Could you check a few things on this model? Use its own coordinates, in mm. A direction names the side the tool comes from. Round coordinates to 2 decimals unless told otherwise and drop trailing zeros. Loops run counter-clockwise (first coordinate to the right, second up) from the corner with the lowest first, then second, coordinate; pieces in that order, holes last. Notation, with made-up numbers: (-20.75, 39) - (-1.75, 39) arc R5 cw to (-1.75, 44) - close; hole circle Ø11 at (46.25, 42). An arc over 180 degrees is marked (long way). Answer as CSV lines item,"result". Start each with the question number.
1) Suppose I cut it at A-A, the plane y = 0.75. Write out the boundary of the cut face in (x, z), then the cut area to 3 significant figures.
2) We'd pull the mould along Z, two halves only. Please class faces 4 (the face through (-1.515, 3.301, 2.597)), 5 (the face through (0, 4, -2.85)), 6 (the face through (-3.25, 5, 0)), 7 (the face through (-3.496, 3.285, 2.049)): pulls with the +Z half, pulls with the -Z half, needs draft (parallel to the pull), parting line crosses it, or undercut.
3) Suppose I cut it at B-B, the plane y = -1. Write out the boundary of the cut face in (x, z).
4) Suppose I cut it at C-C, the plane x = 2.5. Write out the boundary of the cut face in (y, z), then the cut area to 3 significant figures.
5) Suppose I cut it at D-D, the plane z = -0.4. Write out the boundary of the cut face in (x, y), then the cut area to 3 significant figures.
6) Which directions (+Z, -Z, +X, -X, +Y, -Y) give clear straight access to the entire face, cutting with the end or side of a thin tool? Please do faces 1 (the face through (3.504, 3.285, 2.049)), 2 (the face through (0, 2, 0)), 3 (the face through (0.57, 0.5, 0)).
7) I'm going to push flat-ended pins straight in: pin 1 Ø1 at (x, z) = (-0.5, 2.5) entering from +Y; pin 2 Ø0.8 at (x, y) = (1, -1.5) entering from -Z; pin 3 Ø0.8 at (y, z) = (-0.5, 0.5) entering from -X; pin 4 Ø1.5 at (x, z) = (-1.5, 2) entering from +Y. Where does each tip first touch, or does it pass through?
8) Please list where these lines run through material, in increasing order: line 1 along X through (y, z) = (0.25, -2.2); line 2 along Z through (x, y) = (-2.75, 5); line 3 along X through (y, z) = (4.75, -2.1).
```python
from build123d import *
from OCP.BRepFilletAPI import BRepFilletAPI_MakeChamfer

# Parameters (mm, degrees)
CROQUIS2_W              = 7.5
CROQUIS2_H              = 5.7
SALIENTE_EXTRUIR1_DEPTH = 7.2
CROQUIS3_W              = 6.5
CROQUIS3_H              = 4.7
CORTAR_EXTRUIR1_DEPTH   = 5.2
CROQUIS4_W              = 3.6
CROQUIS4_H              = 0.5
CORTAR_EXTRUIR2_DEPTH   = 4.2
CROQUIS5_W              = 1
CROQUIS5_H              = 4.2
CORTAR_EXTRUIR3_DEPTH   = 11.780190165
REDONDEO1_R             = 1
CROQUIS7_W              = 1.4
CROQUIS7_H              = 5.7
CORTAR_EXTRUIR4_DEPTH   = 1
SALIENTE_EXTRUIR2_START = -7.2
CROQUIS6_W              = 0.7
CROQUIS6_H              = 0.7
SALIENTE_EXTRUIR2_DEPTH = 10.7
CHAFL_N1_SIZE           = 0.4
CHAFL_N1_SIZE2          = 0.107179677
CHAFL_N2_SIZE           = 0.4
CHAFL_N2_SIZE2          = 0.107179677
CHAFL_N3_SIZE           = 0.4
CHAFL_N3_SIZE2          = 0.107179677


with BuildPart() as part:
    # Croquis2 → Saliente-Extruir1 (new body)
    with BuildSketch(Plane(origin=(0, 0, 0), x_dir=(1, 0, 0), z_dir=(0, 1, 0))):
        Rectangle(CROQUIS2_W, CROQUIS2_H)
    extrude(amount=SALIENTE_EXTRUIR1_DEPTH)

    # Croquis3 → Cortar-Extruir1 (cut)
    with BuildSketch(Plane(origin=(0, 7.2, 0), x_dir=(1, 0, 0), z_dir=(0, 1, 0))):
        Rectangle(CROQUIS3_W, CROQUIS3_H)
    extrude(amount=-CORTAR_EXTRUIR1_DEPTH, mode=Mode.SUBTRACT)

    # Croquis4 → Cortar-Extruir2 (cut)
    with BuildSketch(Plane(origin=(0, 7.2, 0), x_dir=(1, 0, 0), z_dir=(0, 1, 0))):
        with Locations((0, -2.6)):
            Rectangle(CROQUIS4_W, CROQUIS4_H)
    extrude(amount=-CORTAR_EXTRUIR2_DEPTH, mode=Mode.SUBTRACT)

    # Croquis5 → Cortar-Extruir3 (cut, through all)
    with BuildSketch(Plane(origin=(3.75, 0, 0), x_dir=(0, 0, -1), z_dir=(1, 0, 0))):
        with Locations((-1.85, 5.1)):
            Rectangle(CROQUIS5_W, CROQUIS5_H)
    extrude(amount=-CORTAR_EXTRUIR3_DEPTH, mode=Mode.SUBTRACT)

    # Redondeo1
    # the kernel refuses this fillet: 1 mm, written as the material it adds along each edge
    with BuildSketch(Plane(origin=(1.8, 3, 2.85), x_dir=(0, 1, 0), z_dir=(0, 0, -1)), Plane(origin=(3.75, 3, 2.35), x_dir=(0, 0, -1), z_dir=(-1, 0, 0))) as redondeo1_piece_1:
        with BuildLine():
            CenterArc((REDONDEO1_R, -REDONDEO1_R), REDONDEO1_R, 90, 90)
            Line((0, -REDONDEO1_R), (0, 0))
            Line((0, 0), (REDONDEO1_R, 0))
        make_face()
    extrude(amount=0.5)
    with BuildSketch(Plane(origin=(-1.8, 3, 2.35), x_dir=(1, 0, 0), z_dir=(0, 0, 1)), Plane(origin=(-3.25, 3, 2.35), x_dir=(0, 1, 0), z_dir=(-1, 0, 0))) as redondeo1_piece_2:
        with BuildLine():
            CenterArc((REDONDEO1_R, REDONDEO1_R), REDONDEO1_R, 180, 90)
            Line((0, REDONDEO1_R), (0, 0))
            Line((0, 0), (REDONDEO1_R, 0))
        make_face()
    extrude(amount=0.5)

    # Croquis7 → Cortar-Extruir4 (cut)
    with BuildSketch(Plane.XZ):
        with Locations((-1.27, 0)):
            Rectangle(CROQUIS7_W, CROQUIS7_H)
        with Locations((1.27, 0)):
            Rectangle(CROQUIS7_W, CROQUIS7_H)
    extrude(amount=-CORTAR_EXTRUIR4_DEPTH, mode=Mode.SUBTRACT)

    # Croquis6 → Saliente-Extruir2 (add)
    with BuildSketch(Plane.XZ.offset(SALIENTE_EXTRUIR2_START)):
        with Locations((-1.27, 0.35)):
            Rectangle(CROQUIS6_W, CROQUIS6_H)
        with Locations((1.27, 0.35)):
            Rectangle(CROQUIS6_W, CROQUIS6_H)
    extrude(amount=SALIENTE_EXTRUIR2_DEPTH)

    # Chaflán1: one chamfer whose edges measure the first distance from different faces: ONE call of the kernel's chamfer builder (chamfer() names one face for all edges)
    chafl_n1_edges_1 = [part.edges().sort_by_distance(p)[0] for p in [
        (-0.92, -3.5, 0.35),
    ]]
    chafl_n1_side_1 = [part.faces().sort_by_distance(p)[0] for p in [
        (-0.92, -1.25, 0.35),
    ]]
    chafl_n1_edges_2 = [part.edges().sort_by_distance(p)[0] for p in [
        (-1.27, -3.5, 0.7),
    ]]
    chafl_n1_side_2 = [part.faces().sort_by_distance(p)[0] for p in [
        (-1.27, -1.25, 0.7),
    ]]
    chafl_n1_edges_3 = [part.edges().sort_by_distance(p)[0] for p in [
        (-1.62, -3.5, 0.35),
    ]]
    chafl_n1_side_3 = [part.faces().sort_by_distance(p)[0] for p in [
        (-1.62, -1.25, 0.35),
    ]]
    chafl_n1_edges_4 = [part.edges().sort_by_distance(p)[0] for p in [
        (-1.27, -3.5, 0),
    ]]
    chafl_n1_side_4 = [part.faces().sort_by_distance(p)[0] for p in [
        (-1.27, -1.25, 0),
    ]]
    chafl_n1_edges_5 = [part.edges().sort_by_distance(p)[0] for p in [
        (1.62, -3.5, 0.35),
    ]]
    chafl_n1_side_5 = [part.faces().sort_by_distance(p)[0] for p in [
        (1.62, -1.25, 0.35),
    ]]
    chafl_n1_edges_6 = [part.edges().sort_by_distance(p)[0] for p in [
        (1.27, -3.5, 0.7),
    ]]
    chafl_n1_side_6 = [part.faces().sort_by_distance(p)[0] for p in [
        (1.27, -1.25, 0.7),
    ]]
    chafl_n1_edges_7 = [part.edges().sort_by_distance(p)[0] for p in [
        (0.92, -3.5, 0.35),
    ]]
    chafl_n1_side_7 = [part.faces().sort_by_distance(p)[0] for p in [
        (0.92, -1.25, 0.35),
    ]]
    chafl_n1_edges_8 = [part.edges().sort_by_distance(p)[0] for p in [
        (1.27, -3.5, 0),
    ]]
    chafl_n1_side_8 = [part.faces().sort_by_distance(p)[0] for p in [
        (1.27, -1.25, 0),
    ]]
    chafl_n1 = BRepFilletAPI_MakeChamfer(part.part.solid().wrapped)
    for e in chafl_n1_edges_1:
        chafl_n1.Add(CHAFL_N1_SIZE, CHAFL_N1_SIZE2, e.wrapped, chafl_n1_side_1[0].wrapped)  # the first distance lies on this face
    for e in chafl_n1_edges_2:
        chafl_n1.Add(CHAFL_N1_SIZE, CHAFL_N1_SIZE2, e.wrapped, chafl_n1_side_2[0].wrapped)  # the first distance lies on this face
    for e in chafl_n1_edges_3:
        chafl_n1.Add(CHAFL_N1_SIZE, CHAFL_N1_SIZE2, e.wrapped, chafl_n1_side_3[0].wrapped)  # the first distance lies on this face
    for e in chafl_n1_edges_4:
        chafl_n1.Add(CHAFL_N1_SIZE, CHAFL_N1_SIZE2, e.wrapped, chafl_n1_side_4[0].wrapped)  # the first distance lies on this face
    for e in chafl_n1_edges_5:
        chafl_n1.Add(CHAFL_N1_SIZE, CHAFL_N1_SIZE2, e.wrapped, chafl_n1_side_5[0].wrapped)  # the first distance lies on this face
    for e in chafl_n1_edges_6:
        chafl_n1.Add(CHAFL_N1_SIZE, CHAFL_N1_SIZE2, e.wrapped, chafl_n1_side_6[0].wrapped)  # the first distance lies on this face
    for e in chafl_n1_edges_7:
        chafl_n1.Add(CHAFL_N1_SIZE, CHAFL_N1_SIZE2, e.wrapped, chafl_n1_side_7[0].wrapped)  # the first distance lies on this face
    for e in chafl_n1_edges_8:
        chafl_n1.Add(CHAFL_N1_SIZE, CHAFL_N1_SIZE2, e.wrapped, chafl_n1_side_8[0].wrapped)  # the first distance lies on this face
    add(Compound.cast(chafl_n1.Shape()), mode=Mode.REPLACE)

    # Chaflán2: one chamfer whose edges measure the first distance from different faces: ONE call of the kernel's chamfer builder (chamfer() names one face for all edges)
    chafl_n2_edges_1 = [part.edges().sort_by_distance(p)[0] for p in [
        (-1.27, 7.2, 0.7),
    ]]
    chafl_n2_side_1 = [part.faces().sort_by_distance(p)[0] for p in [
        (-1.27, 4.6, 0.7),
    ]]
    chafl_n2_edges_2 = [part.edges().sort_by_distance(p)[0] for p in [
        (-1.62, 7.2, 0.35),
    ]]
    chafl_n2_side_2 = [part.faces().sort_by_distance(p)[0] for p in [
        (-1.62, 4.6, 0.35),
    ]]
    chafl_n2_edges_3 = [part.edges().sort_by_distance(p)[0] for p in [
        (-1.27, 7.2, 0),
    ]]
    chafl_n2_side_3 = [part.faces().sort_by_distance(p)[0] for p in [
        (-1.27, 4.6, 0),
    ]]
    chafl_n2_edges_4 = [part.edges().sort_by_distance(p)[0] for p in [
        (-0.92, 7.2, 0.35),
    ]]
    chafl_n2_side_4 = [part.faces().sort_by_distance(p)[0] for p in [
        (-0.92, 4.6, 0.35),
    ]]
    chafl_n2 = BRepFilletAPI_MakeChamfer(part.part.solid().wrapped)
    for e in chafl_n2_edges_1:
        chafl_n2.Add(CHAFL_N2_SIZE, CHAFL_N2_SIZE2, e.wrapped, chafl_n2_side_1[0].wrapped)  # the first distance lies on this face
    for e in chafl_n2_edges_2:
        chafl_n2.Add(CHAFL_N2_SIZE, CHAFL_N2_SIZE2, e.wrapped, chafl_n2_side_2[0].wrapped)  # the first distance lies on this face
    for e in chafl_n2_edges_3:
        chafl_n2.Add(CHAFL_N2_SIZE, CHAFL_N2_SIZE2, e.wrapped, chafl_n2_side_3[0].wrapped)  # the first distance lies on this face
    for e in chafl_n2_edges_4:
        chafl_n2.Add(CHAFL_N2_SIZE, CHAFL_N2_SIZE2, e.wrapped, chafl_n2_side_4[0].wrapped)  # the first distance lies on this face
    add(Compound.cast(chafl_n2.Shape()), mode=Mode.REPLACE)

    # Chaflán3: one chamfer whose edges measure the first distance from different faces: ONE call of the kernel's chamfer builder (chamfer() names one face for all edges)
    chafl_n3_edges_1 = [part.edges().sort_by_distance(p)[0] for p in [
        (1.27, 7.2, 0.7),
    ]]
    chafl_n3_side_1 = [part.faces().sort_by_distance(p)[0] for p in [
        (1.27, 4.6, 0.7),
    ]]
    chafl_n3_edges_2 = [part.edges().sort_by_distance(p)[0] for p in [
        (0.92, 7.2, 0.35),
    ]]
    chafl_n3_side_2 = [part.faces().sort_by_distance(p)[0] for p in [
        (0.92, 4.6, 0.35),
    ]]
    chafl_n3_edges_3 = [part.edges().sort_by_distance(p)[0] for p in [
        (1.27, 7.2, 0),
    ]]
    chafl_n3_side_3 = [part.faces().sort_by_distance(p)[0] for p in [
        (1.27, 4.6, 0),
    ]]
    chafl_n3_edges_4 = [part.edges().sort_by_distance(p)[0] for p in [
        (1.62, 7.2, 0.35),
    ]]
    chafl_n3_side_4 = [part.faces().sort_by_distance(p)[0] for p in [
        (1.62, 4.6, 0.35),
    ]]
    chafl_n3 = BRepFilletAPI_MakeChamfer(part.part.solid().wrapped)
    for e in chafl_n3_edges_1:
        chafl_n3.Add(CHAFL_N3_SIZE, CHAFL_N3_SIZE2, e.wrapped, chafl_n3_side_1[0].wrapped)  # the first distance lies on this face
    for e in chafl_n3_edges_2:
        chafl_n3.Add(CHAFL_N3_SIZE, CHAFL_N3_SIZE2, e.wrapped, chafl_n3_side_2[0].wrapped)  # the first distance lies on this face
    for e in chafl_n3_edges_3:
        chafl_n3.Add(CHAFL_N3_SIZE, CHAFL_N3_SIZE2, e.wrapped, chafl_n3_side_3[0].wrapped)  # the first distance lies on this face
    for e in chafl_n3_edges_4:
        chafl_n3.Add(CHAFL_N3_SIZE, CHAFL_N3_SIZE2, e.wrapped, chafl_n3_side_4[0].wrapped)  # the first distance lies on this face
    add(Compound.cast(chafl_n3.Shape()), mode=Mode.REPLACE)


solid = part.part
```
Filled sheet:
1,outline,"(-3.75, -2.85) - (-1.97, -2.85) - (-1.97, 2.85) - (-3.75, 2.85) - close; (-1.62, 0) - (-0.92, 0) - (-0.92, 0.7) - (-1.62, 0.7) - close; (-0.57, -2.85) - (0.57, -2.85) - (0.57, 2.85) - (-0.57, 2.85) - close; (0.92, 0) - (1.62, 0) - (1.62, 0.7) - (0.92, 0.7) - close; (1.97, -2.85) - (3.75, -2.85) - (3.75, 2.85) - (1.97, 2.85) - close"
1,area,"27.8 mm²"
2,face 4,"needs draft"
2,face 5,"pulls with the -Z half"
2,face 6,"undercut"
2,face 7,"undercut"
3,outline,"(-1.62, 0) - (-0.92, 0) - (-0.92, 0.7) - (-1.62, 0.7) - close; (0.92, 0) - (1.62, 0) - (1.62, 0.7) - (0.92, 0.7) - close"
4,outline,"(0, -2.85) - (7.2, -2.85) - (7.2, -2.35) - (2, -2.35) - (2, 2.35) - (7.2, 2.35) - (7.2, 2.85) - (0, 2.85) - close"
4,area,"16.6 mm²"
5,outline,"(-3.75, 0) - (-1.97, 0) - (-1.97, 1) - (-0.57, 1) - (-0.57, 0) - (0.57, 0) - (0.57, 1) - (1.97, 1) - (1.97, 0) - (3.75, 0) - (3.75, 7.2) - (3.25, 7.2) - (3.25, 2) - (-3.25, 2) - (-3.25, 7.2) - (-3.75, 7.2) - close"
5,area,"17.4 mm²"
6,face 1,"+X, -X, +Y"
6,face 2,"+Y"
6,face 3,"+Z, -Z, -Y"
7,pin 1,"y = 3.02"
7,pin 2,"z = 0"
7,pin 3,"x = -1.62"
7,pin 4,"y = 7.2"
8,line 1,"-3.75 to -1.97, -0.57 to 0.57, 1.97 to 3.75"
8,line 2,"-2.85 to -2.35, 2.35 to 2.85"
8,line 3,"-3.75 to -3.25, 3.25 to 3.75"
